from build123d import *

# Parameters (mm, degrees)
SKETCH1_W           = 65
SKETCH1_H           = 95.5
BOSS_EXTRUDE1_DEPTH = 2
SKETCH1_3_W         = 62.5
SKETCH1_3_H         = 92.5
BOSS_EXTRUDE2_DEPTH = 6
SKETCH2_4_W         = 19.6
SKETCH2_4_H         = 19.6
BOSS_EXTRUDE3_DEPTH = 6
CUT_EXTRUDE2_DEPTH  = 39
CUT_EXTRUDE3_DEPTH  = 10
FILLET1_R           = 4
BOSS_EXTRUDE4_DEPTH = 1
SKETCH5_W           = 19.6
SKETCH5_H           = 19.6
CUT_EXTRUDE7_DEPTH  = 4
SKETCH8_W           = 6
SKETCH8_H           = 6
CUT_EXTRUDE8_DEPTH  = 10


with BuildPart() as part:
    # Sketch1 → Boss-Extrude1 (new body)
    with BuildSketch(Plane(origin=(0, 0, 0), x_dir=(1, 0, 0), z_dir=(0, 1, 0))):
        Rectangle(SKETCH1_W, SKETCH1_H)
    extrude(amount=BOSS_EXTRUDE1_DEPTH)

    # Sketch1<3> → Boss-Extrude2 (add)
    with BuildSketch(Plane(origin=(0, 0, 0), x_dir=(1, 0, 0), z_dir=(0, 1, 0))):
        Rectangle(SKETCH1_3_W, SKETCH1_3_H)
    extrude(amount=BOSS_EXTRUDE2_DEPTH)

    # Sketch2<4> → Boss-Extrude3 (add)
    with BuildSketch(Plane(origin=(0, 0, 0), x_dir=(1, 0, 0), z_dir=(0, 1, 0))):
        Rectangle(SKETCH2_4_W, SKETCH2_4_H)
    extrude(amount=BOSS_EXTRUDE3_DEPTH)

    # Sketch2 → Cut-Extrude2 (cut)
    with BuildSketch(Plane(origin=(0, 0, 0), x_dir=(1, 0, 0), z_dir=(0, 1, 0))):
        with BuildLine():
            Line((-7.8, 7.8), (-7.8, -7.8))
            Line((-7.8, -7.8), (7.8, -7.8))
            Line((7.8, -7.8), (7.8, -0.8))
            ThreePointArc((7.8, -0.8), (8.928220211, 1), (7.8, 2.8))
            Line((7.8, 2.8), (7.8, 7.8))
            Line((7.8, 7.8), (-7.8, 7.8))
        make_face()
    extrude(amount=CUT_EXTRUDE2_DEPTH, mode=Mode.SUBTRACT)

    # Sketch3 → Cut-Extrude3 (cut)
    with BuildSketch(Plane(origin=(0, 0, 0), x_dir=(1, 0, 0), z_dir=(0, 1, 0))):
        with BuildLine():
            Line((-30.433287704, 49.156662819), (-34.566712296, 46.343337181))
            Line((-34.566712296, 46.343337181), (-30.346723838, 40.143200294))
            ThreePointArc((-30.346723838, 40.143200294), (-26.873348724, 39.483150817), (-26.213299247, 42.956525932))
            Line((-26.213299247, 42.956525932), (-30.433287704, 49.156662819))
        make_face()
        with BuildLine():
            Line((34.566712296, 46.343337181), (30.433287704, 49.156662819))
            Line((30.433287704, 49.156662819), (26.213299247, 42.956525932))
            ThreePointArc((26.213299247, 42.956525932), (26.873348724, 39.483150817), (30.346723838, 40.143200294))
            Line((30.346723838, 40.143200294), (34.566712296, 46.343337181))
        make_face()
        with BuildLine():
            Line((-30.346723838, -40.143200294), (-34.566712296, -46.343337181))
            Line((-34.566712296, -46.343337181), (-30.433287704, -49.156662819))
            Line((-30.433287704, -49.156662819), (-26.213299247, -42.956525932))
            ThreePointArc((-26.213299247, -42.956525932), (-26.873348724, -39.483150817), (-30.346723838, -40.143200294))
        make_face()
        with BuildLine():
            Line((26.213299247, -42.956525932), (30.433287704, -49.156662819))
            Line((30.433287704, -49.156662819), (34.566712296, -46.343337181))
            Line((34.566712296, -46.343337181), (30.346723838, -40.143200294))
            ThreePointArc((30.346723838, -40.143200294), (26.873348724, -39.483150817), (26.213299247, -42.956525932))
        make_face()
    extrude(amount=CUT_EXTRUDE3_DEPTH, mode=Mode.SUBTRACT)

    # Fillet1
    # the kernel refuses this fillet: 4 mm, written as the material it takes off along each edge
    with BuildSketch(Plane(origin=(-36.876651276, 6, 49.737170606), x_dir=(0, -1, 0), z_dir=(0.5626651276372232, 0, -0.826684918297768)), Plane(origin=(30.346723838, 6, 40.143200294), x_dir=(0, -1, 0), z_dir=(0.5626651276372238, 0, 0.8266849182977677)), Plane(origin=(36.876651276, 6, -49.737170606), x_dir=(0, -1, 0), z_dir=(-0.562665127637224, 0, 0.8266849182977676)), Plane(origin=(-30.346723838, 6, -40.143200294), x_dir=(0, -1, 0), z_dir=(-0.5626651276372242, 0, -0.8266849182977674))) as fillet1_piece_1:
        with BuildLine():
            CenterArc((FILLET1_R, FILLET1_R), FILLET1_R, 180, 90)
            Line((0, FILLET1_R), (0, 0))
            Line((0, 0), (FILLET1_R, 0))
        make_face()
    extrude(amount=11.605353019, mode=Mode.SUBTRACT)
    with BuildSketch(Plane(origin=(-26.213299247, 6, 42.956525932), x_dir=(0, -1, 0), z_dir=(-0.5626651276372243, 0, 0.8266849182977672)), Plane(origin=(34.081582088, 6, 54.516849183), x_dir=(0, -1, 0), z_dir=(-0.5626651276372246, 0, -0.826684918297767)), Plane(origin=(26.213299247, 6, -42.956525932), x_dir=(0, -1, 0), z_dir=(0.5626651276372232, 0, -0.826684918297768)), Plane(origin=(-34.081582088, 6, -54.516849183), x_dir=(0, -1, 0), z_dir=(0.562665127637224, 0, 0.8266849182977676))) as fillet1_piece_2:
        with BuildLine():
            CenterArc((FILLET1_R, FILLET1_R), FILLET1_R, 180, 90)
            Line((0, FILLET1_R), (0, 0))
            Line((0, 0), (FILLET1_R, 0))
        make_face()
    extrude(amount=13.983953251, mode=Mode.SUBTRACT)
    with BuildSketch(Plane(origin=(-28.280011543, 6, 41.549863113), x_dir=(-0.8266849182977704, 0, -0.5626651276372198), z_dir=(-0.5626651276372198, 0, 0.8266849182977704))) as fillet1_piece_3:
        with BuildLine():
            CenterArc((2.5 + FILLET1_R, FILLET1_R), FILLET1_R, 180, 90)
            Line((2.5 + FILLET1_R, 0), (2.5, 0))
            Line((2.5, 0), (2.5, FILLET1_R))
        make_face()
    revolve(axis=Axis((-28.280011543, 6, 41.549863113), (0, -1, 0)), revolution_arc=180, mode=Mode.SUBTRACT)
    with BuildSketch(Plane(origin=(28.280011543, 6, 41.549863113), x_dir=(-0.8266849182977659, 0, 0.5626651276372262), z_dir=(0.5626651276372262, 0, 0.8266849182977659))) as fillet1_piece_4:
        with BuildLine():
            CenterArc((2.5 + FILLET1_R, FILLET1_R), FILLET1_R, 180, 90)
            Line((2.5 + FILLET1_R, 0), (2.5, 0))
            Line((2.5, 0), (2.5, FILLET1_R))
        make_face()
    revolve(axis=Axis((28.280011543, 6, 41.549863113), (0, -1, 0)), revolution_arc=180, mode=Mode.SUBTRACT)
    with BuildSketch(Plane(origin=(28.280011543, 6, -41.549863113), x_dir=(0.826684918297769, 0, 0.5626651276372218), z_dir=(0.5626651276372218, 0, -0.826684918297769))) as fillet1_piece_5:
        with BuildLine():
            CenterArc((2.5 + FILLET1_R, FILLET1_R), FILLET1_R, 180, 90)
            Line((2.5 + FILLET1_R, 0), (2.5, 0))
            Line((2.5, 0), (2.5, FILLET1_R))
        make_face()
    revolve(axis=Axis((28.280011543, 6, -41.549863113), (0, -1, 0)), revolution_arc=180, mode=Mode.SUBTRACT)
    with BuildSketch(Plane(origin=(-28.280011543, 6, -41.549863113), x_dir=(0.8266849182977655, 0, -0.562665127637227), z_dir=(-0.562665127637227, 0, -0.8266849182977655))) as fillet1_piece_6:
        with BuildLine():
            CenterArc((2.5 + FILLET1_R, FILLET1_R), FILLET1_R, 180, 90)
            Line((2.5 + FILLET1_R, 0), (2.5, 0))
            Line((2.5, 0), (2.5, FILLET1_R))
        make_face()
    revolve(axis=Axis((-28.280011543, 6, -41.549863113), (0, -1, 0)), revolution_arc=180, mode=Mode.SUBTRACT)

    # Sketch7 → Boss-Extrude4 (add)
    with BuildSketch(Plane(origin=(0, 0, 0), x_dir=(1, 0, 0), z_dir=(0, 1, 0))):
        with BuildLine():
            Line((7.8, 2.8), (7.8, -0.8))
            ThreePointArc((7.8, -0.8), (8.928220211, 1), (7.8, 2.8))
        make_face()
    extrude(amount=BOSS_EXTRUDE4_DEPTH)

    # Sketch5 → Cut-Extrude7 (cut)
    with BuildSketch(Plane(origin=(0, 6, 0), x_dir=(1, 0, 0), z_dir=(0, 1, 0))):
        Polygon((-21.756286609, -45.25), (21.756286609, -45.25), (30.25, -45.25), (30.25, -34.313210193), (30.25, 34.313210193), (30.25, 45.25), (21.756286609, 45.25), (-21.756286609, 45.25), (-30.25, 45.25), (-30.25, 34.313210193), (-30.25, -34.313210193), (-30.25, -45.25), align=None)
        Rectangle(SKETCH5_W, SKETCH5_H, mode=Mode.SUBTRACT)
    extrude(amount=-CUT_EXTRUDE7_DEPTH, mode=Mode.SUBTRACT)

    # Sketch8 → Cut-Extrude8 (cut)
    with BuildSketch(Plane(origin=(0, 2, 0), x_dir=(1, 0, 0), z_dir=(0, 1, 0))):
        with Locations((6.8, 6.8)):
            Rectangle(SKETCH8_W, SKETCH8_H)
        with Locations((-6.8, 6.8)):
            Rectangle(SKETCH8_W, SKETCH8_H)
        with Locations((-6.8, -6.8)):
            Rectangle(SKETCH8_W, SKETCH8_H)
        with Locations((6.8, -6.8)):
            Rectangle(SKETCH8_W, SKETCH8_H)
    extrude(amount=CUT_EXTRUDE8_DEPTH, mode=Mode.SUBTRACT)


solid = part.part
Verification items for the finished model (mm, model axes). A direction names the side the tool comes from. Give positions to 0.01 mm unless a question says otherwise; leave off trailing zeros. Loops run counter-clockwise (first coordinate to the right, second up) from the corner with the lowest first, then second, coordinate; pieces in that order, holes last. Notation, with made-up numbers: (68, -25.5) - (114, -25.5) arc R14 ccw to (114, -10.5) - close; hole circle Ø7 at (-38.75, 82). An arc over 180 degrees is marked (long way). Write item = value, one per line. Start each with the question number.
Q1. Cross-section at A-A, the plane z = -5. Enter the section's corners in (x, y), and give its area (3 significant figures).
Q2. Cross-section at C-C, the plane x = -19.5. Enter the section's corners in (y, z).
Q3. Depth check by flat-ended pin: P1, Ø3, axis at y = 3, z = -3.5, coming from the +X side; P2, Ø0.6, axis at x = 32, z = 10, coming from the +Y side; P3, Ø1, axis at y = 3.5, z = 8.5, coming from the +X side; P4, Ø1, axis at x = 9, y = 5, coming from the -Z side. Enter the tip coordinate at first touch or a pass-through.
Q4. Mould release check, pull along Z, two halves, no side actions. Record for faces 1 (the face through (-30.852, 3.181, 40.568)), 2 (the face through (27.82, 0.99, 45.32)), 3 (the face through (-30.25, 4, -1)), 4 (the face through (-31.44, 0.99, -41.75)): released by +Z, released by -Z, zero draft, split by the parting line, or undercut.
Q5. Cross-section at D-D, the plane z = 23.5. Enter the section's corners in (x, y), and give its area (3 significant figures).
Q6. Tool access check on faces 5 (the face through (0, 4, 45.25)), 6 (the face through (-31.25, 4, 1)), 7 (the face through (-3.8, 4, -9)), 8 (the face through (31.25, 4, 1)). Record the directions out of +Z, -Z, +X, -X, +Y, -Y that give a thin tool (end or side, any length) a straight path to the whole face; none if there is none.
Q7. Thickness scan on line 1 (Z direction, x = -3.5, y = 5.5); line 2 (X direction, y = 2.25, z = 8.5); line 3 (Z direction, x = 19, y = 4). Record the ranges inside material, lowest first.
Q8. Cross-section at B-B, the plane x = 1.5. Enter the section's corners in (y, z).
Answer key:
q1.outline = (-32.5, 0) - (-7.8, 0) - (-7.8, 2) - (-30.25, 2) - (-30.25, 6) - (-31.25, 6) - (-31.25, 2) - (-32.5, 2) - close; (7.8, 0) - (32.5, 0) - (32.5, 2) - (31.25, 2) - (31.25, 6) - (30.25, 6) - (30.25, 2) - (7.8, 2) - close
q1.area = 107 mm^2
q2.outline = (0, -47.75) - (2, -47.75) - (2, -46.25) - (6, -46.25) - (6, -45.25) - (2, -45.25) - (2, 45.25) - (6, 45.25) - (6, 46.25) - (2, 46.25) - (2, 47.75) - (0, 47.75) - close
q3.P1 = 32.5
q3.P2 = 2
q3.P3 = 31.25
q3.P4 = -46.25
q4.face_1 = released by +Z
q4.face_2 = undercut
q4.face_3 = zero draft
q4.face_4 = released by -Z
q5.outline = (-32.5, 0) - (32.5, 0) - (32.5, 2) - (31.25, 2) - (31.25, 6) - (30.25, 6) - (30.25, 2) - (-30.25, 2) - (-30.25, 6) - (-31.25, 6) - (-31.25, 2) - (-32.5, 2) - close
q5.area = 138 mm^2
q6.face_5 = +X, -X, +Y
q6.face_6 = +Z, -Z, -X, +Y
q6.face_7 = +Y
q6.face_8 = +Z, -Z, +X, +Y
q7.line_1 = -46.25 to -45.25, -9.8 to -7.8, 7.8 to 9.8, 45.25 to 46.25
q7.line_2 = -31.25 to -30.25, -3.8 to 3.8, 30.25 to 31.25
q7.line_3 = -46.25 to -45.25, 45.25 to 46.25
q8.outline = (0, -47.75) - (2, -47.75) - (2, -46.25) - (6, -46.25) - (6, -45.25) - (2, -45.25) - (2, -9.8) - (6, -9.8) - (6, -7.8) - (0, -7.8) - close; (0, 7.8) - (6, 7.8) - (6, 9.8) - (2, 9.8) - (2, 45.25) - (6, 45.25) - (6, 46.25) - (2, 46.25) - (2, 47.75) - (0, 47.75) - close
